The model under review builds one solid part; all positions refer to its coordinate system, in mm. Coordinates: 2 decimals unless noted, no trailing zeros. Write each loop counter-clockwise with the first axis right and the second up, starting at its lowest first coordinate (ties: lowest second). Pieces come first, ordered by that corner, then holes.
1) For line 1 (X direction, y = 1.05, z = 38); line 2 (Z direction, x = -4, y = 1.5); line 3 (Z direction, x = 4.5, y = 0.5), list the stretches that pass through material, from the lowest coordinate up.
2) For P1, Ø0.6, axis at y = 1, z = 36, coming from the +X side, flat-tipped, find the tip position at first contact; note if it passes through.
3) Add section D-D, the plane x = 5. State the section outline as (y, z) points, then the cut area to 3 significant figures.
4) Add section B-B, the plane x = 0. State the section outline as (y, z) points, then the cut area to 3 significant figures.
5) Add section C-C, the plane z = 38. State the section outline as (x, y) points.
6) Add section A-A, the plane z = 0. State the section outline as (x, y) points, then the cut area to 3 significant figures.
from build123d import *

# Parameters (mm, degrees)
SKETCH_2_R      = 21
SKETCH_2_R_2    = 12
SKETCH_2_R_3    = 1.5
EXTRUDE_1_DEPTH = 2
SKETCH_4_W      = 20
SKETCH_4_H      = 25
SKETCH_4_R      = 1.5
EXTRUDE_2_DEPTH = 2
FILLET_1_R      = 10


with BuildPart() as part:
    # 草图2 → 凸台-拉伸1 (new body)
    with BuildSketch(Plane(origin=(0, 0, 0), x_dir=(1, 0, 0), z_dir=(0, 1, 0))):
        with Locations(Location((0, 0, 0), (0, 0, 270))):
            Circle(SKETCH_2_R)
        with Locations(Location((0, 0, 0), (0, 0, 270))):
            Circle(SKETCH_2_R_2, mode=Mode.SUBTRACT)
        with Locations(Location((9.899494937, 9.899494937, 0), (0, 0, 270))):
            Circle(SKETCH_2_R_3, mode=Mode.SUBTRACT)
        with Locations(Location((9.899494937, -9.899494937, 0), (0, 0, 270))):
            Circle(SKETCH_2_R_3, mode=Mode.SUBTRACT)
        with Locations(Location((-9.899494937, -9.899494937, 0), (0, 0, 270))):
            Circle(SKETCH_2_R_3, mode=Mode.SUBTRACT)
        with Locations(Location((-9.899494937, 9.899494937, 0), (0, 0, 270))):
            Circle(SKETCH_2_R_3, mode=Mode.SUBTRACT)
    extrude(amount=EXTRUDE_1_DEPTH)

    # 草图4 → 凸台-拉伸2 (add)
    with BuildSketch(Plane(origin=(0, 2, 0), x_dir=(1, 0, 0), z_dir=(0, 1, 0))):
        with Locations((0, -30.5)):
            Rectangle(SKETCH_4_W, SKETCH_4_H)
        with Locations(Location((-5, -38, 0), (0, 0, 270))):
            Circle(SKETCH_4_R, mode=Mode.SUBTRACT)
        with Locations(Location((5, -38, 0), (0, 0, 270))):
            Circle(SKETCH_4_R, mode=Mode.SUBTRACT)
        with Locations(Location((-5, -28, 0), (0, 0, 270))):
            Circle(SKETCH_4_R, mode=Mode.SUBTRACT)
        with Locations(Location((5, -28, 0), (0, 0, 270))):
            Circle(SKETCH_4_R, mode=Mode.SUBTRACT)
    extrude(amount=-EXTRUDE_2_DEPTH)

    # 圆角1
    fillet_1_edges = [part.edges().sort_by_distance(p)[0] for p in [
        (-10, 1, 18.466185313),
        (10, 1, 18.466185313),
    ]]
    fillet(fillet_1_edges, radius=FILLET_1_R)


solid = part.part
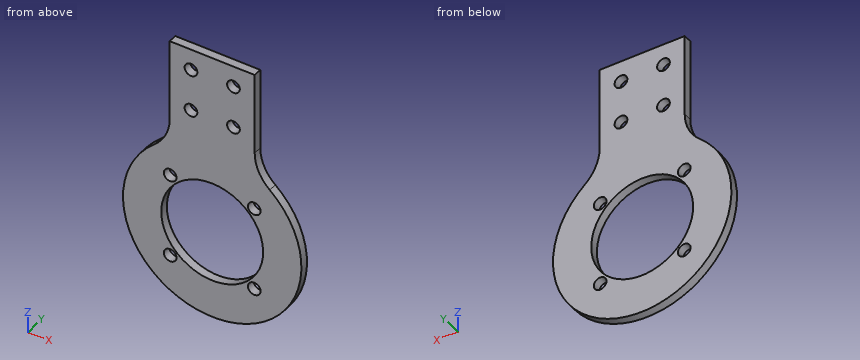
Geometry results:
1. line 1: x = -10 to -6.5, -3.5 to 3.5, 6.5 to 10
1. line 2: z = -20.62 to -11.31, 11.31 to 26.88, 29.12 to 36.88, 39.12 to 43
1. line 3: z = -20.51 to -11.12, 11.12 to 26.59, 29.41 to 36.59, 39.41 to 43
2. P1: stops at x = 10
3. outline: (0, -20.4) - (2, -20.4) - (2, -10.91) - (0, -10.91) - close; (0, 10.91) - (2, 10.91) - (2, 26.5) - (0, 26.5) - close; (0, 29.5) - (2, 29.5) - (2, 36.5) - (0, 36.5) - close; (0, 39.5) - (2, 39.5) - (2, 43) - (0, 43) - close
3. area: 71.2 mm2
4. outline: (0, -21) - (2, -21) - (2, -12) - (0, -12) - close; (0, 12) - (2, 12) - (2, 43) - (0, 43) - close
4. area: 80.0 mm2
5. outline: (-10, 0) - (-6.5, 0) - (-6.5, 2) - (-10, 2) - close; (-3.5, 0) - (3.5, 0) - (3.5, 2) - (-3.5, 2) - close; (6.5, 0) - (10, 0) - (10, 2) - (6.5, 2) - close
6. outline: (-21, 0) - (-12, 0) - (-12, 2) - (-21, 2) - close; (12, 0) - (21, 0) - (21, 2) - (12, 2) - close
6. area: 36.0 mm2
